Verification items for the finished model (mm, model axes). Face numbers are marked on the shaded views. A direction names the side the tool comes from. Give positions to 0.01 mm unless a question says otherwise; leave off trailing zeros. Write each loop counter-clockwise with the first axis right and the second up, starting at its lowest first coordinate (ties: lowest second). Pieces come first, ordered by that corner, then holes. Notation, with made-up numbers: (-23, -12.5) -> (-1, -12.5) arc R12 cw to (-1, -8.5) -> close; hole circle Ø4 at (38.25, 22). An arc over 180 degrees is marked (long way). Write item = value, one per line.
from build123d import *

# Parameters (mm, degrees)
SKETCH5_R           = 3.175
BOSS_EXTRUDE3_DEPTH = 15.875
CHAMFER1_SIZE       = 0.77724
BOSS_EXTRUDE4_DEPTH = 3.96875
SKETCH8_OUTSIDE_W   = 90.54
SKETCH8_OUTSIDE_H   = 92.26
SKETCH8_OUTSIDE_R   = 5.55625
CUT_EXTRUDE3_DEPTH  = 20.84375
CUT_EXTRUDE3_TAPER  = 60
CUT_EXTRUDE4_DEPTH  = 0.254
CIRPATTERN1_COUNT   = 3


with BuildPart() as part:
    # Sketch5 → Boss-Extrude3 (new body)
    with BuildSketch(Plane(origin=(9.921875, 0, 0), x_dir=(0, 0, -1), z_dir=(1, 0, 0))):
        Circle(SKETCH5_R)
    extrude(amount=-BOSS_EXTRUDE3_DEPTH)

    # Chamfer1
    chamfer1_edges = [part.edges().sort_by_distance(p)[0] for p in [
        (9.921875, 0, 3.175),
    ]]
    chamfer(chamfer1_edges, length=CHAMFER1_SIZE)

    # Sketch6 → Boss-Extrude4 (add)
    with BuildSketch(Plane.ZY.offset(5.953125)):
        Polygon((5.55625, 3.207902433), (0, 6.415804866), (-5.55625, 3.207902433), (-5.55625, -3.207902433), (0, -6.415804866), (5.55625, -3.207902433), align=None)
    extrude(amount=BOSS_EXTRUDE4_DEPTH)

    # Sketch8 outside → Cut-Extrude3 (cut, through all)
    with BuildSketch(Plane.ZY.offset(9.921875)):
        Rectangle(SKETCH8_OUTSIDE_W, SKETCH8_OUTSIDE_H)
        Circle(SKETCH8_OUTSIDE_R, mode=Mode.SUBTRACT)
    extrude(amount=-CUT_EXTRUDE3_DEPTH, taper=CUT_EXTRUDE3_TAPER, mode=Mode.SUBTRACT)

    # Sketch12 → Cut-Extrude4 (cut)
    with BuildSketch(Plane.ZY.offset(9.921875)):
        with BuildLine():
            Line((0.1666875, 4.2783125), (0.1666875, 2.3891875))
            ThreePointArc((0.1666875, 2.3891875), (0, 2.2225), (-0.1666875, 2.3891875))
            Line((-0.1666875, 2.3891875), (-0.1666875, 4.2783125))
            ThreePointArc((-0.1666875, 4.2783125), (0, 4.445), (0.1666875, 4.2783125))
        make_face()
    cut_extrude4 = extrude(amount=-CUT_EXTRUDE4_DEPTH, mode=Mode.SUBTRACT)

    # CirPattern1: Cut-Extrude4 ×3 about axis
    cirpattern1_axis = Axis((0, 0, 0), (1, 0, 0))
    for i in range(1, CIRPATTERN1_COUNT):
        add(cut_extrude4.rotate(cirpattern1_axis, i * 360 / CIRPATTERN1_COUNT), mode=Mode.SUBTRACT)


solid = part.part
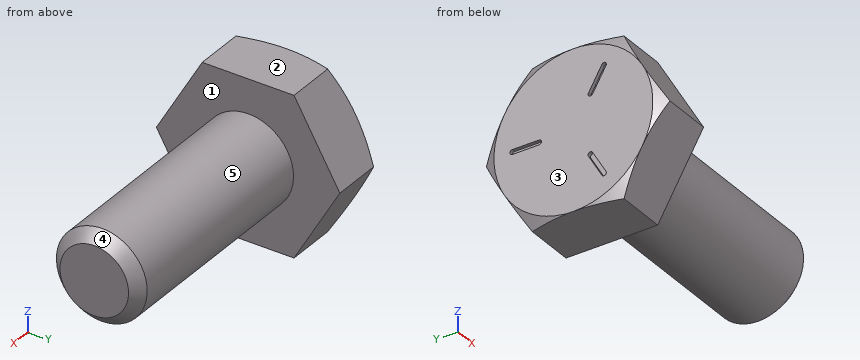
Item 1: Sectioned sample at A-A on x = -4.25. Record the cut outline in (y, z) (3 decimals).
Response values:
outline = circle Ø6.35 at (0, 0)
Item 2: Set-up check for the marked faces 1 and 2: record each of +Z, -Z, +X, -X, +Y, -Y from which the full face is reachable in a straight line by a thin tool's end or side.
Response values:
face_1 = +X
face_2 = +Z, +X, -X, +Y, -Y
Item 3: Go/stop test with flat-tipped pins: P1, Ø2, axis at x = 3.5, y = 2.5, coming from the +Z side; P2, Ø1.5, axis at x = 6, y = 2, coming from the +Z side; P3, Ø1.5, axis at x = 6.5, z = -2.5, coming from the +Y side; P4, Ø3, axis at y = 1, z = -3, coming from the +X side. Record where each tip stops, or that it passes through.
Response values:
P1 = 2.8
P2 = 2.92
P3 = 2.65
P4 = 9.92
Item 4: Mould release check, pull along X, two halves, no side actions. Record for the marked faces 3, 4 and 5: +X half, -X half, draft (parallel to the pull), parting line (faces both ways), or undercut.
Response values:
face_3 = -X half
face_4 = +X half
face_5 = draft
Item 5: Material ranges on line 1 (Y direction, x = 4, z = 0) (3 decimals); line 2 (X direction, y = 3, z = -2); line 3 (Y direction, x = -7.5, z = 2.5), recorded low to high.
Response values:
line_1 = -3.175 to 3.175
line_2 = -9.92 to -5.95
line_3 = -4.97 to 4.97
